The listing builds one solid part. Answer for the finished solid, in the listing's coordinates (mm). Give positions to 0.01 mm unless a question says otherwise; leave off trailing zeros. Loops run counter-clockwise (first coordinate to the right, second up) from the corner with the lowest first, then second, coordinate; pieces in that order, holes last. Notation, with made-up numbers: M -34,2.5 L -7,2.5 A8 cw -7,8.5 Z; hole C 0.5,35.25 d7. An arc over 180 degrees is marked long. One line per item, written item: value. Start each with the question number.
Q1. A cutting plane is placed at C-C, the plane x = 41. Determine the outline of the cut face in (y, z), and give its area (3 significant figures).
Q2. Flat-ended cylindrical pins translate along their axes: pin 1 (1.5 mm diameter, centred on y = 1, z = -124.5, fed in from +X); pin 2 (3 mm diameter, centred on x = 17, z = -155, fed in from +Y); pin 3 (1 mm diameter, centred on x = 107.5, y = 1.5, fed in from -Z). Find the tip coordinate at first contact, or state that the pin passes through.
Q3. A cutting plane is placed at A-A, the plane z = -25. Determine the outline of the cut face in (x, y), and give its area (3 significant figures).
Q4. A cutting plane is placed at B-B, the plane x = 83. Determine the outline of the cut face in (y, z), and give its area (3 significant figures).
Q5. Consider L1, parallel to Z at x = 28.5, y = 1.5; L2, parallel to X at y = 2.4, z = -70; L3, parallel to Z at x = 88.5, y = 0.35. Determine where each line is inside the solid, lowest interval first.
Q6. A cutting plane is placed at D-D, the plane y = 1. State how many separate pieces and enclosed holes the cut face has, and give its area (3 significant figures).
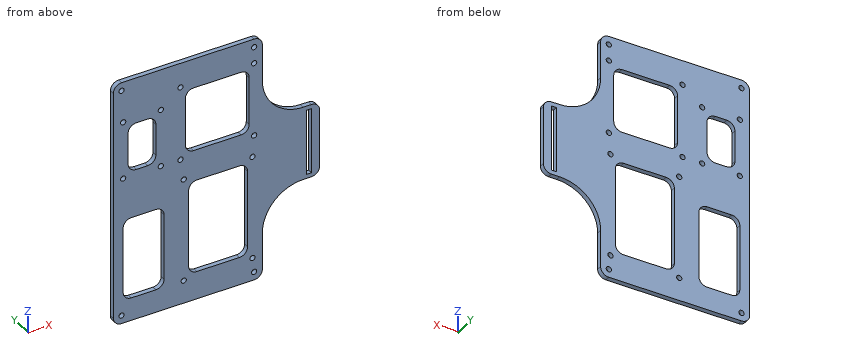
from build123d import *

# Parameters (mm, degrees)
SKETCH1_W           = 138
SKETCH1_H           = 170
BOSS_EXTRUDE1_DEPTH = 3
SKETCH2_R           = 2.1
SKETCH2_W           = 29
SKETCH2_H           = 30
CUT_EXTRUDE1_DEPTH  = 3
SKETCH3_R           = 2.1
CUT_EXTRUDE2_DEPTH  = 219.981734398
SKETCH5_W           = 29
SKETCH5_H           = 35
CUT_EXTRUDE3_DEPTH  = 219.981734398
SKETCH6_R           = 1.6
SKETCH6_W           = 3
SKETCH6_H           = 15
CUT_EXTRUDE4_DEPTH  = 219.981734398
SKETCH9_W           = 29
SKETCH9_H           = 30
BOSS_EXTRUDE2_DEPTH = 3
SKETCH15_W          = 29
SKETCH15_H          = 65
BOSS_EXTRUDE3_DEPTH = 3
SKETCH14_R          = 1.6
SKETCH14_W          = 25
SKETCH14_H          = 50
SKETCH14_W_2        = 36
SKETCH14_H_2        = 57
SKETCH14_W_3        = 39
SKETCH14_H_3        = 39
SKETCH14_W_4        = 17
SKETCH14_H_4        = 29
CUT_EXTRUDE8_DEPTH  = 219.981734398
SKETCH16_W          = 35
SKETCH16_H          = 62.5
SKETCH16_W_2        = 12
SKETCH16_H_2        = 170
CUT_EXTRUDE9_DEPTH  = 219.981734398
SKETCH17_W          = 3
SKETCH17_H          = 40
SKETCH17_W_2        = 91
SKETCH17_H_2        = 10
CUT_EXTRUDE10_DEPTH = 219.981734398
SKETCH18_W          = 10
SKETCH18_H          = 10
BOSS_EXTRUDE4_DEPTH = 3
FILLET5_R           = 5
FILLET6_R           = 25
FILLET7_R           = 5
SKETCH20_R          = 1.6
CUT_EXTRUDE11_DEPTH = 212.3125647
FILLET8_R           = 5


with BuildPart() as part:
    # Sketch1 → Boss-Extrude1 (new body)
    with BuildSketch(Plane(origin=(0, 0, 0), x_dir=(1, 0, 0), z_dir=(0, 1, 0))):
        with Locations((69, 85)):
            Rectangle(SKETCH1_W, SKETCH1_H)
    extrude(amount=BOSS_EXTRUDE1_DEPTH)

    # Sketch2 → Cut-Extrude1 (cut)
    with BuildSketch(Plane(origin=(0, 3, 0), x_dir=(1, 0, 0), z_dir=(0, 1, 0))):
        with Locations(Location((69, 165, 0), (0, 0, 270))):
            Circle(SKETCH2_R)
        with Locations(Location((69, 5, 0), (0, 0, 270))):
            Circle(SKETCH2_R)
        with Locations((14.5, 155)):
            Rectangle(SKETCH2_W, SKETCH2_H)
        with Locations((123.5, 155)):
            Rectangle(SKETCH2_W, SKETCH2_H)
        with Locations((123.5, 15)):
            Rectangle(SKETCH2_W, SKETCH2_H)
        with Locations((14.5, 15)):
            Rectangle(SKETCH2_W, SKETCH2_H)
    extrude(amount=-CUT_EXTRUDE1_DEPTH, mode=Mode.SUBTRACT)

    # Sketch3 → Cut-Extrude2 (cut, through all)
    with BuildSketch(Plane(origin=(0, 3, 0), x_dir=(1, 0, 0), z_dir=(0, 1, 0))):
        with Locations(Location((14, 125, 0), (0, 0, 270))):
            Circle(SKETCH3_R)
        with Locations(Location((14, 45, 0), (0, 0, 270))):
            Circle(SKETCH3_R)
        with Locations(Location((14, 85, 0), (0, 0, 270))):
            Circle(SKETCH3_R)
        with Locations(Location((124, 45, 0), (0, 0, 90))):
            Circle(SKETCH3_R)
        with Locations(Location((124, 125, 0), (0, 0, 90))):
            Circle(SKETCH3_R)
    extrude(amount=-CUT_EXTRUDE2_DEPTH, mode=Mode.SUBTRACT)

    # Sketch5 → Cut-Extrude3 (cut, through all)
    with BuildSketch(Plane(origin=(0, 3, 0), x_dir=(1, 0, 0), z_dir=(0, 1, 0))):
        with Locations((14.5, 122.5)):
            Rectangle(SKETCH5_W, SKETCH5_H)
        with Locations((14.5, 47.5)):
            Rectangle(SKETCH5_W, SKETCH5_H)
    extrude(amount=-CUT_EXTRUDE3_DEPTH, mode=Mode.SUBTRACT)

    # Sketch6 → Cut-Extrude4 (cut, through all)
    with BuildSketch(Plane(origin=(0, 3, 0), x_dir=(1, 0, 0), z_dir=(0, 1, 0))):
        with Locations(Location((131.5, 113, 0), (0, 0, 270))):
            Circle(SKETCH6_R)
        with Locations(Location((131.5, 57, 0), (0, 0, 270))):
            Circle(SKETCH6_R)
        with Locations((131.5, 97.5)):
            Rectangle(SKETCH6_W, SKETCH6_H)
        with Locations((131.5, 72.5)):
            Rectangle(SKETCH6_W, SKETCH6_H)
    extrude(amount=-CUT_EXTRUDE4_DEPTH, mode=Mode.SUBTRACT)

    # Sketch9 → Boss-Extrude2 (add)
    with BuildSketch(Plane(origin=(0, 3, 0), x_dir=(1, 0, 0), z_dir=(0, 1, 0))):
        with Locations((123.5, 155)):
            Rectangle(SKETCH9_W, SKETCH9_H)
        with Locations((123.5, 15)):
            Rectangle(SKETCH9_W, SKETCH9_H)
    extrude(amount=-BOSS_EXTRUDE2_DEPTH)

    # Sketch15 → Boss-Extrude3 (add)
    with BuildSketch(Plane(origin=(0, 3, 0), x_dir=(1, 0, 0), z_dir=(0, 1, 0))):
        with Locations((14.5, 137.5)):
            Rectangle(SKETCH15_W, SKETCH15_H)
        with Locations((14.5, 32.5)):
            Rectangle(SKETCH15_W, SKETCH15_H)
    extrude(amount=-BOSS_EXTRUDE3_DEPTH)

    # Sketch14 → Cut-Extrude8 (cut, through all)
    with BuildSketch(Plane(origin=(0, 3, 0), x_dir=(1, 0, 0), z_dir=(0, 1, 0))):
        with Locations(Location((55, 146, 0), (0, 0, 270))):
            Circle(SKETCH14_R)
        with Locations(Location((97, 146, 0), (0, 0, 270))):
            Circle(SKETCH14_R)
        with Locations(Location((55, 83, 0), (0, 0, 270))):
            Circle(SKETCH14_R)
        with Locations(Location((97, 83, 0), (0, 0, 270))):
            Circle(SKETCH14_R)
        with Locations(Location((53, 70, 0), (0, 0, 270))):
            Circle(SKETCH14_R)
        with Locations(Location((98, 70, 0), (0, 0, 270))):
            Circle(SKETCH14_R)
        with Locations(Location((53, 25, 0), (0, 0, 270))):
            Circle(SKETCH14_R)
        with Locations(Location((98, 25, 0), (0, 0, 270))):
            Circle(SKETCH14_R)
        with Locations(Location((41, 70, 0), (0, 0, 270))):
            Circle(SKETCH14_R)
        with Locations(Location((18, 70, 0), (0, 0, 270))):
            Circle(SKETCH14_R)
        with Locations(Location((18, 35, 0), (0, 0, 270))):
            Circle(SKETCH14_R)
        with Locations(Location((41, 35, 0), (0, 0, 270))):
            Circle(SKETCH14_R)
        with Locations((30.5, 121)):
            Rectangle(SKETCH14_W, SKETCH14_H)
        with Locations((76, 114.5)):
            Rectangle(SKETCH14_W_2, SKETCH14_H_2)
        with Locations((75.5, 47.5)):
            Rectangle(SKETCH14_W_3, SKETCH14_H_3)
        with Locations((29.5, 52.5)):
            Rectangle(SKETCH14_W_4, SKETCH14_H_4)
    extrude(amount=-CUT_EXTRUDE8_DEPTH, mode=Mode.SUBTRACT)

    # Sketch16 → Cut-Extrude9 (cut, through all)
    with BuildSketch(Plane(origin=(0, 3, 0), x_dir=(1, 0, 0), z_dir=(0, 1, 0))):
        with Locations((120.5, 138.75)):
            Rectangle(SKETCH16_W, SKETCH16_H)
        with Locations((120.5, 31.25)):
            Rectangle(SKETCH16_W, SKETCH16_H)
        with Locations((6, 85)):
            Rectangle(SKETCH16_W_2, SKETCH16_H_2)
    extrude(amount=-CUT_EXTRUDE9_DEPTH, mode=Mode.SUBTRACT)

    # Sketch17 → Cut-Extrude10 (cut, through all)
    with BuildSketch(Plane(origin=(0, 3, 0), x_dir=(1, 0, 0), z_dir=(0, 1, 0))):
        with Locations((131.5, 85)):
            Rectangle(SKETCH17_W, SKETCH17_H)
        with Locations((57.5, 165)):
            Rectangle(SKETCH17_W_2, SKETCH17_H_2)
        with Locations((57.5, 5)):
            Rectangle(SKETCH17_W_2, SKETCH17_H_2)
    extrude(amount=-CUT_EXTRUDE10_DEPTH, mode=Mode.SUBTRACT)

    # Sketch18 → Boss-Extrude4 (add)
    with BuildSketch(Plane(origin=(0, 3, 0), x_dir=(1, 0, 0), z_dir=(0, 1, 0))):
        with Locations((17, 85)):
            Rectangle(SKETCH18_W, SKETCH18_H)
    extrude(amount=-BOSS_EXTRUDE4_DEPTH)

    # Fillet5
    fillet5_edges = [part.edges().sort_by_distance(p)[0] for p in [
        (138, 1.5, -62.5),
        (138, 1.5, -107.5),
        (12, 1.5, -160),
        (103, 1.5, -160),
        (12, 1.5, -10),
        (103, 1.5, -10),
    ]]
    fillet(fillet5_edges, radius=FILLET5_R)

    # Fillet6
    fillet6_edges = [part.edges().sort_by_distance(p)[0] for p in [
        (103, 1.5, -62.5),
        (103, 1.5, -107.5),
    ]]
    fillet(fillet6_edges, radius=FILLET6_R)

    # Fillet7
    fillet7_edges = [part.edges().sort_by_distance(p)[0] for p in [
        (18, 1.5, -96),
        (18, 1.5, -146),
        (43, 1.5, -146),
        (43, 1.5, -96),
    ]]
    fillet(fillet7_edges, radius=FILLET7_R)

    # Sketch20 → Cut-Extrude11 (cut, through all)
    with BuildSketch(Plane(origin=(0, 3, 0), x_dir=(1, 0, 0), z_dir=(0, 1, 0))):
        with Locations(Location((17, 155, 0), (0, 0, 270))):
            Circle(SKETCH20_R)
        with Locations(Location((98, 155, 0), (0, 0, 270))):
            Circle(SKETCH20_R)
        with Locations(Location((17, 15, 0), (0, 0, 270))):
            Circle(SKETCH20_R)
        with Locations(Location((98, 15, 0), (0, 0, 270))):
            Circle(SKETCH20_R)
    extrude(amount=-CUT_EXTRUDE11_DEPTH, mode=Mode.SUBTRACT)

    # Fillet8
    fillet8_edges = [part.edges().sort_by_distance(p)[0] for p in [
        (56, 1.5, -28),
        (56, 1.5, -67),
        (95, 1.5, -67),
        (95, 1.5, -28),
        (38, 1.5, -38),
        (21, 1.5, -38),
        (21, 1.5, -67),
        (38, 1.5, -67),
        (58, 1.5, -86),
        (58, 1.5, -143),
        (94, 1.5, -143),
        (94, 1.5, -86),
    ]]
    fillet(fillet8_edges, radius=FILLET8_R)


solid = part.part
Answer block:
1. outline: M 0,-160 L 3,-160 L 3,-145 L 0,-145 Z; M 0,-97 L 3,-97 L 3,-71.6 L 0,-71.6 Z; M 0,-68.4 L 3,-68.4 L 3,-36.6 L 0,-36.6 Z; M 0,-33.4 L 3,-33.4 L 3,-10 L 0,-10 Z
1. area: 287 mm^2
2. pin 1: x = 104.58
2. pin 2: through
2. pin 3: z = -118.94
3. outline: M 12,0 L 51.4,0 L 51.4,3 L 12,3 Z; M 54.6,0 L 96.4,0 L 96.4,3 L 54.6,3 Z; M 99.6,0 L 103,0 L 103,3 L 99.6,3 Z
3. area: 254 mm^2
4. outline: M 0,-160 L 3,-160 L 3,-143 L 0,-143 Z; M 0,-86 L 3,-86 L 3,-67 L 0,-67 Z; M 0,-28 L 3,-28 L 3,-10 L 0,-10 Z
4. area: 162 mm^2
5. L1: -160 to -146, -96 to -67, -38 to -10
5. L2: 12 to 16.4, 19.6 to 39.4, 42.6 to 51.4, 54.6 to 96.4, 99.6 to 130, 133 to 138
5. L3: -160 to -143, -86 to -67, -28 to -10
6. separate pieces: 1
6. enclosed holes: 21
6. area: 9,980 mm^2
